from build123d import *

# Parameters (mm, degrees)
BOSS_EXTRUDE1_DEPTH      = 609.6
BOSS_EXTRUDE1_DEPTH_BACK = 609.6
SKETCH3_W                = 38.1
SKETCH3_H                = 25.4
SKETCH3_W_2              = 31.75
SKETCH3_H_2              = 19.05
SKETCH6_R                = 6.35
CUT_EXTRUDE1_DEPTH       = 611.426262951


with BuildPart() as part:
    # Sketch3 → Boss-Extrude1 (new, two sides: drawn at the far end of the back side and taken through both)
    with BuildSketch(Plane.XY.offset(-BOSS_EXTRUDE1_DEPTH_BACK)):
        Rectangle(SKETCH3_W, SKETCH3_H)
        Rectangle(SKETCH3_W_2, SKETCH3_H_2, mode=Mode.SUBTRACT)
    extrude(amount=BOSS_EXTRUDE1_DEPTH + BOSS_EXTRUDE1_DEPTH_BACK)

    # Sketch6 → Cut-Extrude1 (cut, through all)
    with BuildSketch(Plane(origin=(0, 12.7, 0), x_dir=(1, 0, 0), z_dir=(0, 1, 0))):
        with Locations(Location((-4.7625, -390.525, 0), (0, 0, 270))):
            Circle(SKETCH6_R)
        with Locations(Location((-4.7625, -422.275, 0), (0, 0, 270))):
            Circle(SKETCH6_R)
        with Locations(Location((-4.7625, 422.275, 0), (0, 0, 270))):
            Circle(SKETCH6_R)
        with Locations(Location((-4.7625, 390.525, 0), (0, 0, 270))):
            Circle(SKETCH6_R)
    extrude(amount=-CUT_EXTRUDE1_DEPTH, mode=Mode.SUBTRACT)


solid = part.part
Model file for the job. Use its own axes, mm. A direction names the side the tool comes from. Give positions to 0.01 mm unless a question says otherwise; leave off trailing zeros. Write each loop counter-clockwise with the first axis right and the second up, starting at its lowest first coordinate (ties: lowest second). Pieces come first, ordered by that corner, then holes. Notation, with made-up numbers: (17.25, 33) - (21.25, 33) arc R24 ccw to (21.25, 57) - close; hole circle Ø3 at (-31, -30.5). An arc over 180 degrees is marked (long way). Answer as CSV lines item,"result".
1. Band-saw the part on A-A (z = 123). Write the cut outline in (x, y) (3 decimals), and give its area (3 significant figures).
Responses:
outline,"(-19.05, -12.7) - (19.05, -12.7) - (19.05, 12.7) - (-19.05, 12.7) - close; hole (-15.875, -9.525) - (15.875, -9.525) - (15.875, 9.525) - (-15.875, 9.525) - close"
area,"363 mm2"
2. Band-saw the part on B-B (y = -1.25). Write the cut outline in (x, z) (3 decimals), and give its area (3 significant figures).
Responses:
outline,"(-19.05, -609.6) - (-15.875, -609.6) - (-15.875, 609.6) - (-19.05, 609.6) - close; (15.875, -609.6) - (19.05, -609.6) - (19.05, 609.6) - (15.875, 609.6) - close"
area,"7,740 mm2"
3. Pin check, flat tip, straight feed: pin 1 (11.5 mm diameter, centred on x = -4.76, z = -390.52, fed in from -Y). Stop position of the tip, or through.
Responses:
pin 1,"passes through"
4. 3-axis set-ups, long thin cutter, end or side, ignore diameter. For faces 1 (the face through (0, -11, 609.6)), 2 (the face through (0, -9.525, -9)): which of +Z, -Z, +X, -X, +Y, -Y reach the whole face in a straight line?
Responses:
face 1,"+Z, +X, -X, +Y, -Y"
face 2,"+Z, -Z"
5. Drill centre lines: L1, parallel to Y at x = 7, z = -451 (3 decimals); L2, parallel to X at y = -0.25, z = 129 (3 decimals). Where is each one in solid material? Low to high. Write a range as [from, to].
Responses:
L1,"y = [-12.7, -9.525], [9.525, 12.7]"
L2,"x = [-19.05, -15.875], [15.875, 19.05]"
6. Two-plate mould, pull along Y, no slides. Class faces 3 (the face through (19.05, 0, -9)), 4 (the face through (0, -12.7, -9)), 5 (the face through (0, 12.7, -9)), 6 (the face through (15.875, 0, -9)): +Y half, -Y half, draft (parallel to the pull), parting line (faces both ways), or undercut.
Responses:
face 3,"draft"
face 4,"-Y half"
face 5,"+Y half"
face 6,"undercut"
